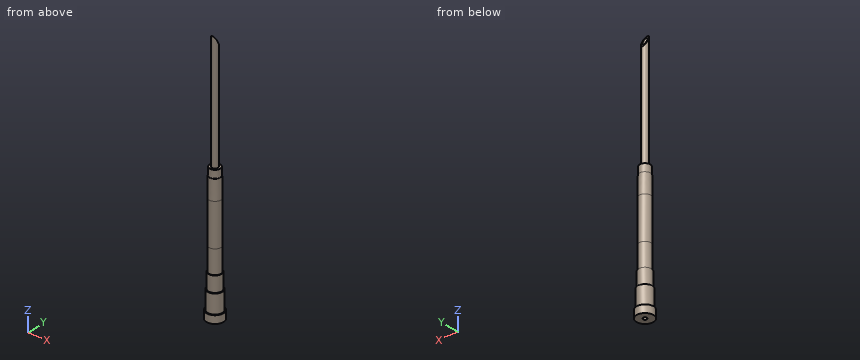
```python
from build123d import *

# Parameters (mm, degrees)
SKETCH1_R           = 5.510734027
BOSS_EXTRUDE1_DEPTH = 5
SKETCH2_R           = 4.80322663
BOSS_EXTRUDE2_DEPTH = 12
SKETCH3_R           = 4.165391046
BOSS_EXTRUDE3_DEPTH = 10
SKETCH4_R           = 3.833295876
BOSS_EXTRUDE4_DEPTH = 15
SKETCH5_R           = 3.610443511
BOSS_EXTRUDE5_DEPTH = 40
SKETCH6_R           = 3.404861597
BOSS_EXTRUDE6_DEPTH = 5
DRAFT3_ANGLE        = 1
SKETCH7_R           = 1.999677314
BOSS_EXTRUDE7_DEPTH = 80
SKETCH8_R           = 1.320990831
CUT_EXTRUDE1_DEPTH  = 170
SKETCH9_W           = 6.196430892
SKETCH9_H           = 6.69100276
BOSS_EXTRUDE8_DEPTH = 5
CUT_EXTRUDE3_DEPTH  = 40


# Read off the part's stored shape, not the designer's step: Draft1
with BuildPart() as part:
    # Sketch1 → Boss-Extrude1 (new body)
    with BuildSketch(Plane.XY):
        Circle(SKETCH1_R)
    extrude(amount=BOSS_EXTRUDE1_DEPTH)

    # Sketch2 → Boss-Extrude2 (add)
    with BuildSketch(Plane.XY.offset(5)):
        Circle(SKETCH2_R)
    extrude(amount=BOSS_EXTRUDE2_DEPTH)

    # Sketch3 → Boss-Extrude3 (add)
    with BuildSketch(Plane.XY.offset(17)):
        Circle(SKETCH3_R)
    extrude(amount=BOSS_EXTRUDE3_DEPTH)

    # Sketch4 → Boss-Extrude4 (add)
    with BuildSketch(Plane.XY.offset(27)):
        Circle(SKETCH4_R)
    extrude(amount=BOSS_EXTRUDE4_DEPTH)

    # Sketch5 → Boss-Extrude5 (add)
    with BuildSketch(Plane.XY.offset(42)):
        Circle(SKETCH5_R)
    extrude(amount=BOSS_EXTRUDE5_DEPTH)

    # Draft1 outline → Draft1 (revolve)
    with BuildSketch(Plane.XZ):
        Polygon((3.833295876, 42), (3.833295876, 69.232796586), (3.610443511, 82), (3.610443511, 42), align=None)
    revolve(axis=Axis((0, 0, 0), (0, 0, 1)))

    # Sketch6 → Boss-Extrude6 (add)
    with BuildSketch(Plane.XY.offset(82)):
        Circle(SKETCH6_R)
    extrude(amount=BOSS_EXTRUDE6_DEPTH)

    # Draft3
    draft3_faces = [part.faces().sort_by_distance(p)[0] for p in [
        (-3.404861597, 0, 84.5),
    ]]
    draft(draft3_faces, Plane.XY.offset(87), DRAFT3_ANGLE)

    # Sketch7 → Boss-Extrude7 (add)
    with BuildSketch(Plane.XY.offset(87)):
        Circle(SKETCH7_R)
    extrude(amount=BOSS_EXTRUDE7_DEPTH)

    # Sketch8 → Cut-Extrude1 (cut)
    with BuildSketch(Plane.XY.offset(167)):
        Circle(SKETCH8_R)
    extrude(amount=-CUT_EXTRUDE1_DEPTH, mode=Mode.SUBTRACT)

    # Sketch9 → Boss-Extrude8 (add)
    with BuildSketch(Plane.XY.offset(167)):
        with Locations((-0.356570781, -0.45222472)):
            Rectangle(SKETCH9_W, SKETCH9_H)
    extrude(amount=BOSS_EXTRUDE8_DEPTH)

    # Sketch10 → Cut-Extrude3 (cut)
    with BuildSketch(Plane(origin=(2.741644665, 0, 0), x_dir=(0, 0, -1), z_dir=(1, 0, 0))):
        Polygon((-152.074864923, 3.565905239), (-141.864160289, 3.91336171), (-152.717774104, 10.240072861), (-183.049805068, 3.30023825), (-173.245812896, -7.716844209), align=None)
    extrude(amount=-CUT_EXTRUDE3_DEPTH, mode=Mode.SUBTRACT)


solid = part.part
```
CAD build for the part. Positions are in the model's coordinates, mm. Round coordinates to 2 decimals unless told otherwise and drop trailing zeros. Loops run counter-clockwise (first coordinate to the right, second up) from the corner with the lowest first, then second, coordinate; pieces in that order, holes last. Notation, with made-up numbers: M 42.5,45 L 89.5,45 A12 ccw 89.5,52 Z; hole C 69.25,6 d9. An arc over 180 degrees is marked long. Use a Markdown table: item, result. Add a question column.
(1) Cut at B-B (z = 116.5). Give the cut face in (x, y), and give its area (3 significant figures).
(2) Flat gauge pins, fed straight in: pin 1 (5 mm diameter, centred on x = 2, y = 3.5, fed in from +Z); pin 2 (3 mm diameter, centred on x = -0.5, y = 0, fed in from +Z); pin 3 (3 mm diameter, centred on x = 1.5, z = 78, fed in from -Y). Where does each tip first touch, or does it go through?
(3) Drill centre lines: line 1 (Y direction, x = 0, z = 109.5); line 2 (Y direction, x = 0, z = 42.5). Where is each one in solid material? Low to high.
(4) Cut at A-A (z = 21). Give the cut face in (x, y), and give its area (3 significant figures).
Geometry says:
| question | item | result |
|---|---|---|
| 1 | outline | C 0,0 d4; hole C 0,0 d2.64 |
| 1 | area | 7.08 mm² |
| 2 | pin 1 | stops at z = 156.86 |
| 2 | pin 2 | stops at z = 161.58 |
| 2 | pin 3 | stops at y = -3.69 |
| 3 | line 1 | y = -2 to -1.32, 1.32 to 2 |
| 3 | line 2 | y = -3.83 to -1.32, 1.32 to 3.83 |
| 4 | outline | C 0,0 d8.33; hole C 0,0 d2.64 |
| 4 | area | 49.0 mm² |
